The model under review builds one solid part; all positions refer to its coordinate system, in mm. A direction names the side the tool comes from. Coordinates: 2 decimals unless noted, no trailing zeros. Write each loop counter-clockwise with the first axis right and the second up, starting at its lowest first coordinate (ties: lowest second). Pieces come first, ordered by that corner, then holes.
```python
from build123d import *

# Parameters (mm, degrees)
PAD_DEPTH       = 14
SKETCH001_R     = 1.5
POCKET_DEPTH    = 91.604738
FILLET_R        = 6
PAD001_DEPTH    = 14
SKETCH003_W     = 12
SKETCH003_H     = 8.899188
POCKET001_DEPTH = 4.5
FILLET001_R     = 3
CHAMFER_SIZE    = 1


with BuildPart() as part:
    # Sketch → Pad (new body)
    with BuildSketch(Plane.XZ):
        Polygon((20, -3), (20, 3), (-20, 3), (-20, -3), (-6.5, -3), (-6.5, 0), (6.5, 0), (6.5, -3), align=None)
    extrude(amount=PAD_DEPTH)

    # Sketch001 (on DatumPlane) → Pocket (cut, through all)
    with BuildSketch(Plane(origin=(0, 0, 3), x_dir=(-1, 0, 0), z_dir=(0, 0, 1))):
        with Locations((14, 7)):
            Circle(SKETCH001_R)
    pocket = extrude(amount=-POCKET_DEPTH, mode=Mode.SUBTRACT)

    # Mirrored: Pocket across Sketch001 V_Axis
    add(pocket.mirror(Plane(origin=(0, 0, 3), x_dir=(0, 0, 1), z_dir=(-1, 0, 0))), mode=Mode.SUBTRACT)

    # Fillet
    fillet_edges = [part.edges().sort_by_distance(p)[0] for p in [
        (-20, -14, 0),
        (20, -14, 0),
        (20, 0, 0),
        (-20, 0, 0),
    ]]
    fillet(fillet_edges, radius=FILLET_R)

    # Sketch002 → Pad001 (join)
    with BuildSketch(Plane.XZ):
        Polygon((-14, 3), (-11, 6), (11, 6), (14, 3), align=None)
    extrude(amount=PAD001_DEPTH)

    # Sketch003 (on DatumPlane) → Pocket001 (cut, symmetric)
    with BuildSketch(Plane(origin=(0, -7, 0), x_dir=(1, 0, 0), z_dir=(0, 1, 0))):
        with Locations((14, -7.449594)):
            Rectangle(SKETCH003_W, SKETCH003_H)
    pocket001 = extrude(amount=POCKET001_DEPTH, both=True, mode=Mode.SUBTRACT)

    # Mirrored001: Pocket001 across Sketch003 V_Axis
    add(pocket001.mirror(Plane(origin=(0, -7, 0), x_dir=(0, 1, 0), z_dir=(1, 0, 0))), mode=Mode.SUBTRACT)

    # Fillet001
    fillet001_edges = [part.edges().sort_by_distance(p)[0] for p in [
        (-8, -11.5, 4.5),
        (8, -11.5, 4.5),
        (-8, -2.5, 4.5),
        (8, -2.5, 4.5),
    ]]
    fillet(fillet001_edges, radius=FILLET001_R)

    # Chamfer
    chamfer_edges = [part.edges().sort_by_distance(p)[0] for p in [
        (-15.06066, -5.93934, 3),
        (12.5, -7, 3),
    ]]
    chamfer(chamfer_edges, length=CHAMFER_SIZE)


solid = part.part
```
Item 1: Take a section at A-A, the plane y = -7. Write out the cut boundary in (x, z).
Solved:
outline: (-20, -3) - (-15.5, -3) - (-15.5, 2) - (-16.5, 3) - (-20, 3) - close; (-12.5, -3) - (-6.5, -3) - (-6.5, 0) - (6.5, 0) - (6.5, -3) - (12.5, -3) - (12.5, 2) - (11.5, 3) - (8, 3) - (8, 6) - (-8, 6) - (-8, 3) - (-11.5, 3) - (-12.5, 2) - close; (15.5, -3) - (20, -3) - (20, 3) - (16.5, 3) - (15.5, 2) - close
Item 2: Take a section at D-D, the plane y = -4. Write out the cut boundary in (x, z).
Solved:
outline: (-19.66, -3) - (-6.5, -3) - (-6.5, 0) - (6.5, 0) - (6.5, -3) - (19.66, -3) - (19.66, 3) - (8.4, 3) - (8.4, 6) - (-8.4, 6) - (-8.4, 3) - (-19.66, 3) - close
Item 3: Machinability: for faces 1 (the face through (-13, -1, 4)), 2 (the face through (-17, -7, 3)), 3 (the face through (-6.5, -7, -2)), 4 (the face through (8.86, -10.6, 4.48)), which of the approach directions +Z, -Z, +X, -X, +Y, -Y give a long, thin tool a straight path to every point of the face, cutting with its end or side? Answer none if there is none.
Solved:
face 1: +Z, -X, +Y, -Y
face 2: +Z, -X
face 3: -Z, +Y, -Y
face 4: +Z, +X
Item 4: Take a section at C-C, the plane x = 3. Write out the cut boundary in (y, z).
Solved:
outline: (-14, 0) - (0, 0) - (0, 6) - (-14, 6) - close
Item 5: Take a section at B-B, the plane z = 0.5. Write out the cut boundary in (x, y).
Solved:
outline: (-20, -8) arc R6 ccw to (-14, -14) - (14, -14) arc R6 ccw to (20, -8) - (20, -6) arc R6 ccw to (14, 0) - (-14, 0) arc R6 ccw to (-20, -6) - close; hole circle Ø3 at (-14, -7); hole circle Ø3 at (14, -7)
Item 6: For pin 1 (2.5 mm diameter, centred on x = -13, z = 5, fed in from -Y); pin 2 (1.8 mm diameter, centred on x = -14, y = -7, fed in from +Z); pin 3 (3.5 mm diameter, centred on x = 11.5, y = -9, fed in from +Z); pin 4 (0.9 mm diameter, centred on y = -7, z = 4.5, fed in from +X), all flat-tipped, find the tip position at first contact; note any pin that passes through.
Solved:
pin 1: stops at y = -14
pin 2: passes through
pin 3: stops at z = 3
pin 4: stops at x = 8
Item 7: To check wall thickness, follow line 1 along Y through (x, z) = (-14, -0.1); line 2 along X through (y, z) = (-7, -1); line 3 along X through (y, z) = (-6.5, -1.5). State the ranges of each line that lie inside material, in increasing order.
Solved:
line 1: y = -14 to -8.5, -5.5 to 0
line 2: x = -20 to -15.5, -12.5 to -6.5, 6.5 to 12.5, 15.5 to 20
line 3: x = -20 to -15.41, -12.59 to -6.5, 6.5 to 12.59, 15.41 to 20
